```python
from build123d import *

# Parameters (mm, degrees)
BOSS_EXTRUDE1_DEPTH = 6
SKETCH2_R           = 8.5
BOSS_EXTRUDE2_DEPTH = 34
BOSS_EXTRUDE3_DEPTH = 6
SKETCH4_R           = 6.75
CUT_EXTRUDE1_DEPTH  = 55
SKETCH5_R           = 2.25
CUT_EXTRUDE2_DEPTH  = 13
SKETCH9_R           = 1.75
CUT_EXTRUDE5_DEPTH  = 57.497787567
FILLET1_R           = 2
CHAMFER4_SIZE       = 2


with BuildPart() as part:
    # Sketch1 → Boss-Extrude1 (new body)
    with BuildSketch(Plane.XY):
        with BuildLine():
            Line((-12, 0), (-12, -14))
            Line((-12, -14), (-20, -14))
            Line((-20, -14), (-20, -20))
            Line((-20, -20), (-12, -20))
            Line((-12, -20), (12, -20))
            Line((12, -20), (20, -20))
            Line((20, -20), (20, -14))
            Line((20, -14), (12, -14))
            Line((12, -14), (12, 0))
            ThreePointArc((12, 0), (0, 12), (-12, 0))
        make_face()
    extrude(amount=BOSS_EXTRUDE1_DEPTH)

    # Sketch2 → Boss-Extrude2 (add)
    with BuildSketch(Plane.XY.offset(6)):
        Circle(SKETCH2_R)
    extrude(amount=BOSS_EXTRUDE2_DEPTH)

    # Sketch3 → Boss-Extrude3 (add)
    with BuildSketch(Plane.XY.offset(40)):
        with BuildLine():
            Line((-12, 0), (-12, -14))
            Line((-12, -14), (-20, -14))
            Line((-20, -14), (-20, -20))
            Line((-20, -20), (20, -20))
            Line((20, -20), (20, -14))
            Line((20, -14), (12, -14))
            Line((12, -14), (12, 0))
            ThreePointArc((12, 0), (0, 12), (-12, 0))
        make_face()
    extrude(amount=BOSS_EXTRUDE3_DEPTH)

    # Sketch4 → Cut-Extrude1 (cut, through all)
    with BuildSketch(Plane.XY.offset(46)):
        Circle(SKETCH4_R)
    extrude(amount=-CUT_EXTRUDE1_DEPTH, mode=Mode.SUBTRACT)

    # Sketch5 → Cut-Extrude2 (cut)
    with BuildSketch(Plane.XZ.offset(20)):
        with Locations((-5, 43)):
            Circle(SKETCH5_R)
        with Locations((5, 43)):
            Circle(SKETCH5_R)
        with Locations((-5, 3)):
            Circle(SKETCH5_R)
        with Locations((5, 3)):
            Circle(SKETCH5_R)
    extrude(amount=-CUT_EXTRUDE2_DEPTH, mode=Mode.SUBTRACT)

    # Sketch9 → Cut-Extrude5 (cut, through all)
    with BuildSketch(Plane(origin=(0, -14, 0), x_dir=(1, 0, 0), z_dir=(0, 1, 0))):
        with Locations(Location((15, -43, 0), (0, 0, 270))):
            Circle(SKETCH9_R)
        with Locations(Location((-15, -43, 0), (0, 0, 270))):
            Circle(SKETCH9_R)
        with Locations(Location((15, -3, 0), (0, 0, 270))):
            Circle(SKETCH9_R)
        with Locations(Location((-15, -3, 0), (0, 0, 270))):
            Circle(SKETCH9_R)
    extrude(amount=-CUT_EXTRUDE5_DEPTH, mode=Mode.SUBTRACT)

    # Fillet1
    fillet1_edges = [part.edges().sort_by_distance(p)[0] for p in [
        (20, -17, 0),
        (-20, -17, 0),
        (20, -17, 6),
        (-20, -17, 40),
        (20, -17, 40),
        (-20, -17, 46),
        (20, -17, 46),
        (-20, -17, 6),
    ]]
    fillet(fillet1_edges, radius=FILLET1_R)

    # Chamfer4
    chamfer4_edges = [part.edges().sort_by_distance(p)[0] for p in [
        (-12, -7, 0),
        (0, 12, 0),
        (12, -7, 0),
        (12, -7, 46),
        (0, 12, 46),
        (-12, -7, 46),
    ]]
    chamfer(chamfer4_edges, length=CHAMFER4_SIZE)


solid = part.part
```
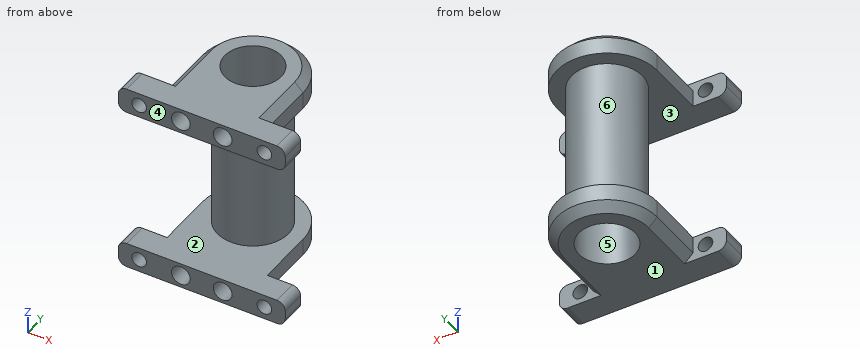
Can you work these out from the model? Positions are in its coordinate system, mm. Face numbers are marked on the shaded views. A direction names the side the tool comes from. Coordinates: 2 decimals unless noted, no trailing zeros. Loops run counter-clockwise (first coordinate to the right, second up) from the corner with the lowest first, then second, coordinate; pieces in that order, holes last. Notation, with made-up numbers: (41.25, 67.25) -> (66.25, 67.25) arc R6 cw to (66.25, 74.25) -> close; hole circle Ø4 at (-27, 52.5). An arc over 180 degrees is marked (long way). Put each result on its own line as item: value. Start each with the question number.
Q1. I want a section at D-D (x = -15). Write out the boundary of the cut face in (y, z).
Q2. For the marked faces 5 and 6, which set-ups out of +Z, -Z, +X, -X, +Y, -Y let a thin tool reach every point of the face, with its end or its side?
Q3. Thinking about a two-plate mould opening in Z: for the marked faces 1, 2, 3 and 4, which applies, pulls with the +Z half, pulls with the -Z half, needs draft (parallel to the pull), parting line crosses it, or undercut?
Q4. If I drill on line 1 (Z direction, x = 5, y = -15); line 2 (Z direction, x = -4.5, y = 8.5); line 3 (Z direction, x = 14, y = -17.5), over which ranges is the centre line in solid material (lowest first)? Write a range as [from, to].
Q5. I want a section at B-B (z = 3). Write out the boundary of the cut face in (x, y), plus the area to 3 significant figures.
Q6. I want a section at C-C (x = 0). Write out the boundary of the cut face in (y, z).
Q7. I'm going to push flat-ended pins straight in: P1, Ø3, axis at y = -4.5, z = 3.5, coming from the +X side; P2, Ø1.8, axis at x = -16.5, z = 44, coming from the +Y side; P3, Ø6, axis at x = 5, z = 43, coming from the +Y side. Where does each tip first touch, or does it pass through?
Q8. I want a section at A-A (y = -17). Count the separate pieces of the cut face and the enclosed holes in it, plus the area to 3 significant figures.
Taken from the geometry:
1. outline: (-20, 0) -> (-14, 0) -> (-14, 1.25) -> (-20, 1.25) -> close; (-20, 4.75) -> (-14, 4.75) -> (-14, 6) -> (-20, 6) -> close; (-20, 40) -> (-14, 40) -> (-14, 41.25) -> (-20, 41.25) -> close; (-20, 44.75) -> (-14, 44.75) -> (-14, 46) -> (-20, 46) -> close
2. face 5: +Z, -Z
2. face 6: none
3. face 1: pulls with the -Z half
3. face 2: undercut
3. face 3: undercut
3. face 4: needs draft
4. line 1: z = [0, 0.75], [5.25, 6], [40, 40.75], [45.25, 46]
4. line 2: z = [0, 6], [40, 46]
4. line 3: z = [0, 1.56], [4.44, 6], [40, 41.56], [44.44, 46]
5. outline: (-20, -20) -> (-16.75, -20) -> (-16.75, -14) -> (-20, -14) -> close; (-13.25, -20) -> (-7.25, -20) -> (-7.25, -7) -> (-2.75, -7) -> (-2.75, -20) -> (2.75, -20) -> (2.75, -7) -> (7.25, -7) -> (7.25, -20) -> (13.25, -20) -> (13.25, -14) -> (12, -14) -> (12, 0) arc R12 ccw to (-12, 0) -> (-12, -14) -> (-13.25, -14) -> close; (16.75, -20) -> (20, -20) -> (20, -14) -> (16.75, -14) -> close; hole circle Ø13.5 at (0, 0)
5. area: 500 mm2
6. outline: (-20, 0) -> (-6.75, 0) -> (-6.75, 46) -> (-20, 46) -> (-20, 40) -> (-8.5, 40) -> (-8.5, 6) -> (-20, 6) -> close; (6.75, 0) -> (10, 0) -> (12, 2) -> (12, 6) -> (8.5, 6) -> (8.5, 40) -> (12, 40) -> (12, 44) -> (10, 46) -> (6.75, 46) -> close
7. P1: stops at x = 12
7. P2: stops at y = -14
7. P3: stops at y = 11.83
8. separate pieces: 2
8. enclosed holes: 8
8. area: 371 mm2
